Geometry check sheet. Reference: the model listing, model coordinates, mm. Face numbers are marked on the shaded views. Coordinates: 2 decimals unless noted, no trailing zeros. Loops run counter-clockwise (first coordinate to the right, second up) from the corner with the lowest first, then second, coordinate; pieces in that order, holes last. Notation, with made-up numbers: (53, -21.75) - (85, -21.75) arc R34 ccw to (85, 12.25) - close; hole circle Ø5 at (2, 53.25). An arc over 180 degrees is marked (long way). Write item = value, one per line. Start each with the question number.
from build123d import *

# Parameters (mm, degrees)
SKETCH_1_R      = 2.55
SKETCH_1_R_2    = 3.05
EXTRUDE_1_DEPTH = 9
FILLET_1_R      = 5


with BuildPart() as part:
    # 草图1 → 凸台-拉伸1 (new body)
    with BuildSketch(Plane.XY):
        Polygon((-54.053450796, 27.320514858), (5.802955665, 27.320514858), (-28.018037849, -17.774143161), align=None)
        with Locations((-40.197044335, 19.320514858)):
            Circle(SKETCH_1_R, mode=Mode.SUBTRACT)
        with Locations((-27.148108815, -3.280904448)):
            Circle(SKETCH_1_R, mode=Mode.SUBTRACT)
        with Locations((-10.197044335, 19.320514858)):
            Circle(SKETCH_1_R, mode=Mode.SUBTRACT)
        with Locations((-24.197044335, 12.320514858)):
            Circle(SKETCH_1_R_2, mode=Mode.SUBTRACT)
    extrude(amount=EXTRUDE_1_DEPTH)

    # 圆角1
    fillet_1_edges = [part.edges().sort_by_distance(p)[0] for p in [
        (-54.053450796, 27.320514858, 4.5),
        (5.802955665, 27.320514858, 4.5),
        (-28.018037849, -17.774143161, 4.5),
    ]]
    fillet(fillet_1_edges, radius=FILLET_1_R)


solid = part.part
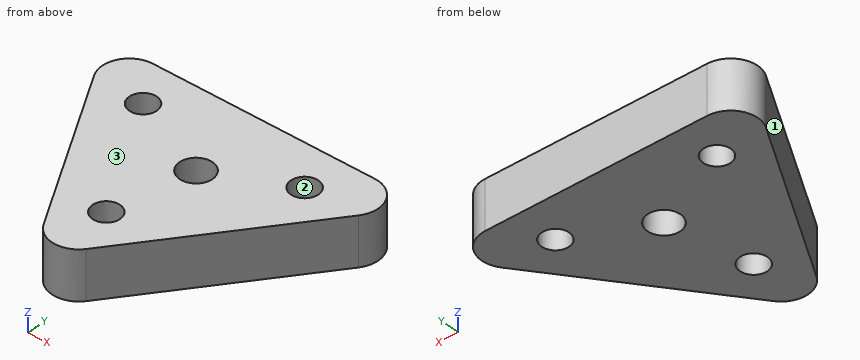
(1) Draft check along X on the marked faces 1, 2 and 3. Enter one of: pulls with the +X half, pulls with the -X half, needs draft (parallel to the pull), parting line crosses it, or undercut.
(2) Sectioned sample at A-A on y = 13. Enter the section's corners in (x, z), plus the area to 3 significant figures.
(3) Depth check by flat-ended pin: pin 1 (3 mm diameter, centred on y = -0.5, z = 1, fed in from +X); pin 2 (1.5 mm diameter, centred on y = 11, z = 6, fed in from -X); pin 3 (3 mm diameter, centred on x = -39, z = 6.5, fed in from -Y). Enter the tip coordinate at first touch or a pass-through.
(4) Sectioned sample at D-D on x = -25.5. Enter the section's corners in (y, z).
(5) Sectioned sample at B-B on x = -11. Enter the section's corners in (y, z).
(6) Sectioned sample at C-C on z = 7.5. Enter the section's corners in (x, y), plus the area to 3 significant figures.
(7) Scan lines: line 1 (X direction, y = 19.5, z = 7.75); line 2 (X direction, y = 18, z = 1.75); line 3 (Y direction, x = -40, z = 7.5). Record each from-to range of solid material in increasing order.
Working result:
q1.face_1 = pulls with the -X half
q1.face_2 = undercut
q1.face_3 = needs draft
q2.outline = (-45.79, 0) - (-27.17, 0) - (-27.17, 9) - (-45.79, 9) - close; (-21.22, 0) - (-4.94, 0) - (-4.94, 9) - (-21.22, 9) - close
q2.area = 314 mm2
q3.pin_1 = -13.94
q3.pin_2 = -45.06
q3.pin_3 = -1.35
q4.outline = (-13.31, 0) - (-5.23, 0) - (-5.23, 9) - (-13.31, 9) - close; (-1.34, 0) - (9.56, 0) - (9.56, 9) - (-1.34, 9) - close; (15.08, 0) - (27.32, 0) - (27.32, 9) - (15.08, 9) - close
q5.outline = (4.92, 0) - (16.9, 0) - (16.9, 9) - (4.92, 9) - close; (21.74, 0) - (27.32, 0) - (27.32, 9) - (21.74, 9) - close
q6.outline = (-49.72, 19.82) - (-31.8, -11.22) arc R5 ccw to (-23.47, -11.72) - (-0.2, 19.32) arc R5 ccw to (-4.2, 27.32) - (-45.39, 27.32) arc R5 ccw to start; hole circle Ø5.1 at (-40.2, 19.32); hole circle Ø5.1 at (-27.15, -3.28); hole circle Ø6.1 at (-24.2, 12.32); hole circle Ø5.1 at (-10.2, 19.32)
q6.area = 1,210 mm2
q7.line_1 = -49.54 to -42.74, -37.65 to -12.74, -7.65 to -0.07
q7.line_2 = -48.67 to -42.38, -38.02 to -12.38, -8.02 to -1.19
q7.line_3 = 2.98 to 16.78, 21.86 to 27.32
